Geometry check sheet. Reference: the model listing, model coordinates, mm. Face numbers are marked on the shaded views. A direction names the side the tool comes from. Coordinates: 2 decimals unless noted, no trailing zeros. Order: outer loops, then holes, each group sorted by start corner. A loop starts at its lowest first (then second) coordinate and runs counter-clockwise, first axis right, second up. Notation, with made-up numbers: M -7.5,-7.75 L 38.5,-7.75 A14 cw 38.5,16.25 Z; hole C 84,-14 d3. An arc over 180 degrees is marked long. One line per item, written item: value. Start each with the question number.
1) Sectioned sample at A-A, the plane y = -127. Enter the section's corners in (x, z).
2) Thickness scan on L1, parallel to X at y = -127, z = -1.25; L2, parallel to X at y = -167, z = -3; L3, parallel to Y at x = -10, z = -3. Record the ranges inside material, lowest first. Write a range as from..to.
3) Access from +Z, -Z, +X, -X, +Y, -Y to the whole of each face (thin tool, end or side, straight path). Record for the marked faces 3 and 4.
4) Draft check along X on the marked faces 1 and 2. Enter one of: pulls with the +X half, pulls with the -X half, needs draft (parallel to the pull), parting line crosses it, or undercut.
5) Sectioned sample at D-D, the plane y = -167. Enter the section's corners in (x, z), then the cut area to 3 significant figures.
6) Go/stop test with flat-tipped pins: P1, Ø4, axis at x = -22.5, y = -144.5, coming from the +Z side; P2, Ø5, axis at x = -17.5, z = -2.5, coming from the +Y side; P3, Ø3, axis at x = 0, y = 8, coming from the +Z side; P4, Ø11, axis at x = 14.5, y = -7, coming from the -Z side. Record where each tip stops, or that it passes through.
7) Sectioned sample at C-C, the plane x = -20. Enter the section's corners in (y, z).
8) Sectioned sample at B-B, the plane y = -37.5. Enter the section's corners in (x, z), then the cut area to 3 significant figures.
```python
from build123d import *

# Parameters (mm, degrees)
SKETCH1_W               = 12
SKETCH1_H               = 30
SKETCH1_R               = 1.65
SKETCH1_R_2             = 2.5
BOSS_EXTRUDE1_DEPTH     = 6.35
FILLET1_R               = 6
FILLET2_R               = 6
FILLET3_R               = 20
SKETCH2_R               = 1.65
CUT_EXTRUDE1_DEPTH      = 10
CUT_EXTRUDE3_DEPTH      = 5
BOSS_EXTRUDE3_DEPTH     = 5
CHAMFER2_SIZE           = 5
FILLET5_R               = 5
SKETCH6_R               = 1.65
CUT_EXTRUDE4_DEPTH      = 178.83791075
CUT_EXTRUDE5_DEPTH      = 178.83791075
CUT_EXTRUDE5_DEPTH_BACK = 2
FILLET6_R               = 3
SKETCH8_W               = 40
SKETCH8_H               = 60
SKETCH8_R               = 1.65
BOSS_EXTRUDE4_DEPTH     = 6.35
FILLET7_R               = 10


with BuildPart() as part:
    # Sketch1 → Boss-Extrude1 (new body)
    # profile 1 of 2: a face of its own
    with BuildSketch(Plane.XY):
        Polygon((6, 15), (6, -15), (6, -175), (31, -175), (31, 15), align=None)
    # profile 2 of 2: a face of its own
    with BuildSketch(Plane.XY):
        Rectangle(SKETCH1_W, SKETCH1_H)
        with Locations((0, -8)):
            Circle(SKETCH1_R, mode=Mode.SUBTRACT)
        Circle(SKETCH1_R_2, mode=Mode.SUBTRACT)
        with Locations((0, 8)):
            Circle(SKETCH1_R, mode=Mode.SUBTRACT)
    extrude(amount=BOSS_EXTRUDE1_DEPTH)

    # Fillet1
    fillet1_edges = [part.edges().sort_by_distance(p)[0] for p in [
        (6, -15, 3.175),
    ]]
    fillet(fillet1_edges, radius=FILLET1_R)
    fillet1_2_edges = [part.edges().sort_by_distance(p)[0] for p in [
        (-6, -15, 3.175),
    ]]
    fillet(fillet1_2_edges, radius=FILLET1_R - 0.0001)  # a hair under: the kernel refuses the full size

    # Fillet2
    fillet2_edges = [part.edges().sort_by_distance(p)[0] for p in [
        (-6, 15, 3.175),
    ]]
    fillet(fillet2_edges, radius=FILLET2_R)

    # Fillet3
    fillet3_edges = [part.edges().sort_by_distance(p)[0] for p in [
        (31, 15, 3.175),
    ]]
    fillet(fillet3_edges, radius=FILLET3_R)

    # Sketch2 → Cut-Extrude1 (cut)
    with BuildSketch(Plane.XY.offset(6.35)):
        with Locations((14, -167)):
            Circle(SKETCH2_R)
        with Locations((14, -127)):
            Circle(SKETCH2_R)
    extrude(amount=-CUT_EXTRUDE1_DEPTH, mode=Mode.SUBTRACT)

    # Sketch3 → Cut-Extrude3 (cut)
    with BuildSketch(Plane.XY.offset(6.35)):
        Polygon((31, -175), (31, -80), (6, -55), (6, -175), align=None)
    extrude(amount=-CUT_EXTRUDE3_DEPTH, mode=Mode.SUBTRACT)

    # Sketch5 → Boss-Extrude3 (add)
    with BuildSketch(Plane(origin=(0, 0, 0), x_dir=(-1, 0, 0), z_dir=(0, 0, -1))):
        Polygon((-6, -175), (-6, -55), (-31, -80), (-31, -175), align=None)
    extrude(amount=BOSS_EXTRUDE3_DEPTH)

    # Chamfer2
    chamfer2_edges = [part.edges().sort_by_distance(p)[0] for p in [
        (18.5, -67.5, 1.35),
        (18.5, -67.5, 0),
    ]]
    chamfer(chamfer2_edges, length=CHAMFER2_SIZE - 0.0001)  # a hair under: the kernel refuses the full size

    # Fillet5
    fillet5_edges = [part.edges().sort_by_distance(p)[0] for p in [
        (18.5, -74.570926391, 1.35),
        (18.5, -60.429073609, 0),
    ]]
    fillet(fillet5_edges, radius=FILLET5_R)

    # Sketch6 → Cut-Extrude4 (cut, through all)
    with BuildSketch(Plane.XY.offset(1.35)):
        with Locations((14, -127)):
            Circle(SKETCH6_R)
        with Locations((14, -167)):
            Circle(SKETCH6_R)
    extrude(amount=-CUT_EXTRUDE4_DEPTH, mode=Mode.SUBTRACT)

    # Sketch7 → Cut-Extrude5 (cut, two sides: drawn at the far end of the back side and taken through both)
    with BuildSketch(Plane.XY.offset(1.35).offset(-CUT_EXTRUDE5_DEPTH_BACK)):
        Polygon((-175.7227113, 75.782237154), (6, -105.940474145), (20.142135624, -120.082609769), (20.142135624, -86.828079155), (6, -72.685943532), (-175.7227113, 109.036767768), (-689.712157123, 109.036767768), (-689.712157123, 75.782237154), align=None)
    extrude(amount=CUT_EXTRUDE5_DEPTH + CUT_EXTRUDE5_DEPTH_BACK, mode=Mode.SUBTRACT)

    # Fillet6
    fillet6_edges = [part.edges().sort_by_distance(p)[0] for p in [
        (20.142135624, -86.828079155, 0.35),
        (20.142135624, -120.082609769, 0.35),
    ]]
    fillet(fillet6_edges, radius=FILLET6_R)

    # Sketch8 → Boss-Extrude4 (add)
    with BuildSketch(Plane.XY.offset(1.35)):
        with Locations((-14, -145)):
            Rectangle(SKETCH8_W, SKETCH8_H)
        with Locations((-27.03159011, -127)):
            Circle(SKETCH8_R, mode=Mode.SUBTRACT)
        with Locations((-27.03159011, -167)):
            Circle(SKETCH8_R, mode=Mode.SUBTRACT)
    extrude(amount=-BOSS_EXTRUDE4_DEPTH)

    # Fillet7
    fillet7_edges = [part.edges().sort_by_distance(p)[0] for p in [
        (6, -115, -1.825),
        (31, -175, -1.825),
        (-34, -175, -1.825),
        (-34, -115, -1.825),
    ]]
    fillet(fillet7_edges, radius=FILLET7_R)


solid = part.part
```
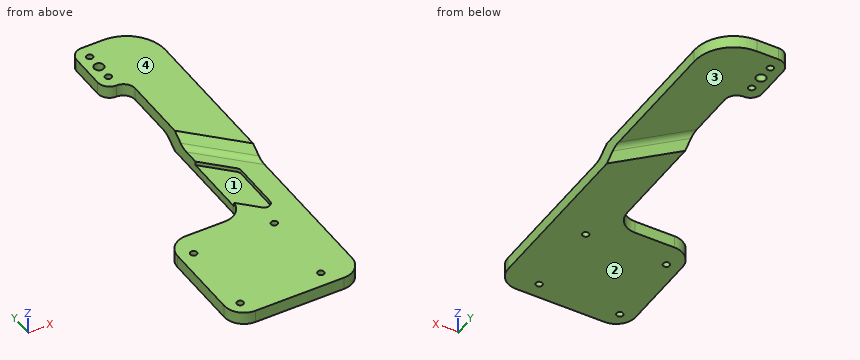
Final values:
1. outline: M -34,-5 L -28.68,-5 L -28.68,1.35 L -34,1.35 Z; M -25.38,-5 L 12.35,-5 L 12.35,1.35 L -25.38,1.35 Z; M 15.65,-5 L 31,-5 L 31,1.35 L 15.65,1.35 Z
2. L1: x = -34..-28.68, -25.38..12.35, 15.65..31
2. L2: x = -33.8..-28.68, -25.38..12.35, 15.65..30.8
2. L3: y = -175..-115
3. face 3: -Z, +X, +Y
3. face 4: +Z, +X, -X, +Y, -Y
4. face 1: undercut
4. face 2: needs draft
5. outline: M -33.8,-5 L -28.68,-5 L -28.68,1.35 L -33.8,1.35 Z; M -25.38,-5 L 12.35,-5 L 12.35,1.35 L -25.38,1.35 Z; M 15.65,-5 L 30.8,-5 L 30.8,1.35 L 15.65,1.35 Z
5. area: 368 mm^2
6. P1: stops at z = 1.35
6. P2: stops at y = -115
6. P3: passes through
6. P4: stops at z = 0
7. outline: M -175,-5 L -115,-5 L -115,1.35 L -175,1.35 Z
8. outline: M 6,0 L 31,0 L 31,6.35 L 6,6.35 Z
8. area: 159 mm^2
